Input: part model. Units: mm. Frame: model coordinates. Face numbers are marked on the shaded views. Coordinates: 2 decimals unless noted, no trailing zeros. Write each loop counter-clockwise with the first axis right and the second up, starting at its lowest first coordinate (ties: lowest second). Pieces come first, ordered by that corner, then holes. Notation, with made-up numbers: (20.25, 88) -> (60.25, 88) arc R18 cw to (60.25, 110) -> close; hole circle Ø7 at (26.25, 83). An arc over 180 degrees is marked (long way). Use one line per item in the form item = value. Start each with the question number.
(1) First-contact query: pin 1 (5 mm diameter, centred on x = -0.5, y = -2, fed in from -Z); pin 2 (3 mm diameter, centred on y = -6, z = 3, fed in from +X); pin 3 (3 mm diameter, centred on y = 5.5, z = 3, fed in from +X); pin 4 (3 mm diameter, centred on y = 7, z = 2, fed in from +X). Flat tips, straight axial feed; report the tip coordinate or a pass-through.
(2) Cut plane A-A on y = 0. Return the cut outline in (x, z).
(3) Pull-direction query (Y, two-part tool) for the marked faces 1, 2 and 3; classes: released by +Y, released by -Y, zero draft, split by the parting line, or undercut.
(4) Cut plane C-C on z = 0.55. Return the cut outline in (x, y).
(5) Cut plane D-D on x = 7.5. Return the cut outline in (y, z), plus the area to 3 significant figures.
(6) Ray query, line 1 along Y through (x, z) = (0, 1.2); line 2 along Z through (x, y) = (7.75, -1); line 3 along Y through (x, z) = (-3.75, 1.25). Return the intervals inside material, ascending.
Autodesk Inventor part; units mm, degrees
ref_plane "YZ Plane" through (0, 0, 0) normal (1, 0, 0) x (0, 1, 0)
ref_plane "XZ Plane" through (0, 0, 0) normal (0, 1, 0) x (-1, 0, 0)
ref_plane "XY Plane" through (0, 0, 0) normal (0, 0, 1) x (1, 0, 0)
sketch "スケッチ1" plane through (0, 0, 0) normal (0, 0, 1) x (1, 0, 0)
  circle A0 centre (0, 0) radius 6
  circle A1 centre (0, 0) radius 5
  dimension "d0" = 12
  dimension "d1" = 10
extrude "押し出し1" add sketch "スケッチ1" along normal blind 5
chamfer "面取り1" distance 0.5 angle 45 1 edges at (-6, 0, 5)
sketch "スケッチ2" plane through (0, 0, 0) normal (0, 0, -1) x (-1, 0, 0)
  circle A0 centre (0, 0) radius 9
  circle A1 centre (0, 0) radius 5
  dimension "d7" = 18
extrude "押し出し2" add sketch "スケッチ2" against normal blind 1
properties part number "オイレスw5f10-12a" material "アセタール樹脂、黒"
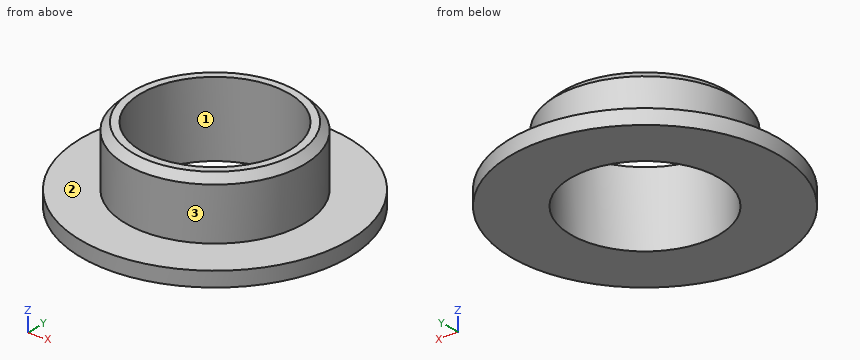
Values:
q1.pin_1 = through
q1.pin_2 = 3.97
q1.pin_3 = 4.47
q1.pin_4 = 6.81
q2.outline = (-9, 0) -> (-5, 0) -> (-5, 5) -> (-5.5, 5) -> (-6, 4.5) -> (-6, 1) -> (-9, 1) -> close; (5, 0) -> (9, 0) -> (9, 1) -> (6, 1) -> (6, 4.5) -> (5.5, 5) -> (5, 5) -> close
q3.face_1 = undercut
q3.face_2 = zero draft
q3.face_3 = split by the parting line
q4.outline = circle Ø18 at (0, 0); hole circle Ø10 at (0, 0)
q5.outline = (-4.97, 0) -> (4.97, 0) -> (4.97, 1) -> (-4.97, 1) -> close
q5.area = 9.95 mm2
q6.line_1 = -6 to -5, 5 to 6
q6.line_2 = 0 to 1
q6.line_3 = -4.68 to -3.31, 3.31 to 4.68
